The drawing under review shows one solid part. Ordinate dimensions are in mm from its lowest x, y, z. Give positions to 0.01 mm unless a question says otherwise; leave off trailing zeros. Loops run counter-clockwise (first coordinate to the right, second up) from the corner with the lowest first, then second, coordinate; pieces in that order, holes last. Notation, with made-up numbers: (-23, 8) - (19, 8) arc R12 cw to (19, 16) - close; hole circle Ø3 at (17, 57.5). An arc over 180 degrees is marked (long way). One line per item, written item: value. Start each with the question number.
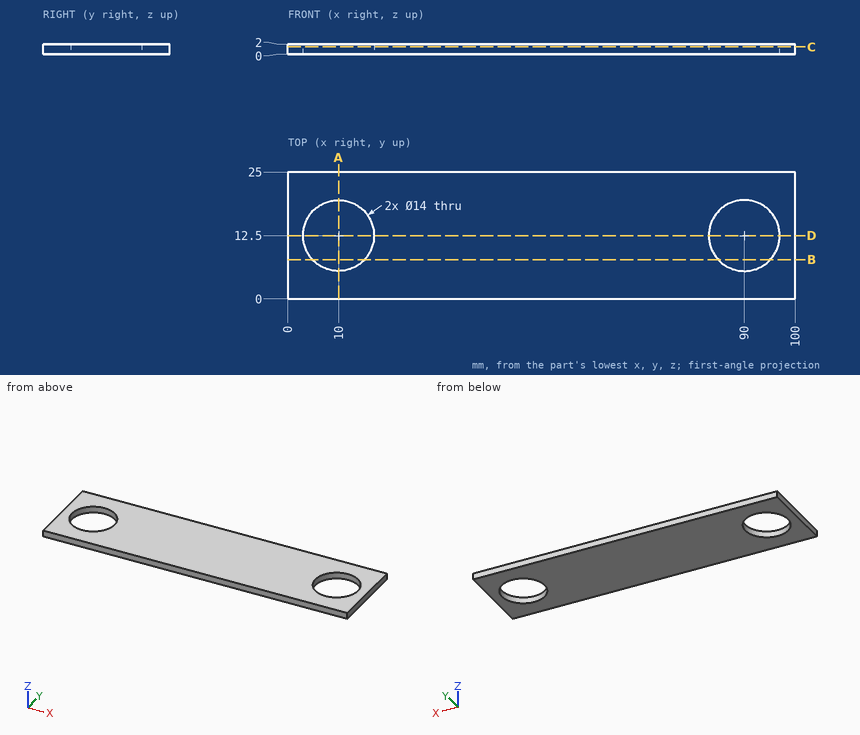
(1) Take a section at B-B on y = 7.75. State the section outline as (x, z) points.
(2) Take a section at A-A on x = 10. State the section outline as (y, z) points.
(3) Take a section at D-D on y = 12.5. State the section outline as (x, z) points.
(4) For pin 1 Ø11 at (x, y) = (10, 12.5) entering from +Z, flat-tipped, find the tip position at first contact; note if it passes through.
(5) To check wall thickness, follow L1, parallel to Y at x = 90, z = 1.45; L2, parallel to X at y = 15.5, z = 0.1; L3, parallel to Y at x = 91, z = 1.45. State the ranges of each line that lie inside material, in increasing order. Write a range as from..to.
(6) Take a section at C-C on z = 1.45. State the section outline as (x, y) points.
Here are the results:
1. outline: (0, 0) - (4.86, 0) - (4.86, 2) - (0, 2) - close; (15.14, 0) - (84.86, 0) - (84.86, 2) - (15.14, 2) - close; (95.14, 0) - (100, 0) - (100, 2) - (95.14, 2) - close
2. outline: (0, 0) - (5.5, 0) - (5.5, 2) - (0, 2) - close; (19.5, 0) - (25, 0) - (25, 2) - (19.5, 2) - close
3. outline: (0, 0) - (3, 0) - (3, 2) - (0, 2) - close; (17, 0) - (83, 0) - (83, 2) - (17, 2) - close; (97, 0) - (100, 0) - (100, 2) - (97, 2) - close
4. pin 1: through
5. L1: 0..5.5, 19.5..25
5. L2: 0..3.68, 16.32..83.68, 96.32..100
5. L3: 0..5.57, 19.43..25
6. outline: (0, 0) - (100, 0) - (100, 25) - (0, 25) - close; hole circle Ø14 at (10, 12.5); hole circle Ø14 at (90, 12.5)
